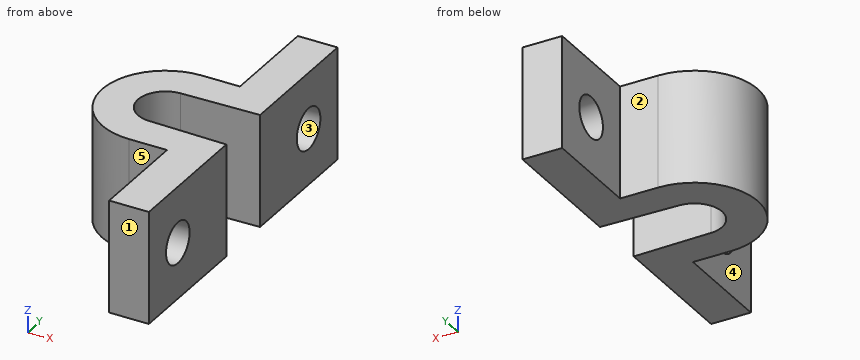
```python
from build123d import *

# Parameters (mm, degrees)
F1_DEPTH = 13
F2_R     = 2.375
F3_DEPTH = 4.6


with BuildPart() as f1:
    # F0 (on Top) → F1 (new body)
    with BuildSketch(Plane.XY):
        with BuildLine():
            Line((-4.6, -19), (0, -19))
            Line((0, -19), (0, -3.4))
            Line((0, -3.4), (-9.075746, -3.184099))
            ThreePointArc((-9.075746, -3.184099), (-12.185, 0), (-9.075746, 3.184099))
            Line((-9.075746, 3.184099), (0, 3.4))
            Line((0, 3.4), (0, 19))
            Line((0, 19), (-4.6, 19))
            Line((-4.6, 19), (-4.6, 7.34))
            Line((-4.6, 7.34), (-9, 7.34))
            ThreePointArc((-9, 7.34), (-16.34, 0), (-9, -7.34))
            Line((-9, -7.34), (-4.6, -7.34))
            Line((-4.6, -7.34), (-4.6, -19))
        make_face()
    extrude(amount=F1_DEPTH)

    # F2 (on Right) → F3 (cut, through all)
    with BuildSketch(Plane.YZ):
        with Locations((-13.17, 6.5)):
            Circle(F2_R)
        with Locations((13.17, 6.5)):
            Circle(F2_R)
    extrude(amount=-F3_DEPTH, mode=Mode.SUBTRACT)


solid = f1.part
```
Model file for the job. Use its own axes, mm. Face numbers are marked on the shaded views. A direction names the side the tool comes from. Give positions to 0.01 mm unless a question says otherwise; leave off trailing zeros. Write each loop counter-clockwise with the first axis right and the second up, starting at its lowest first coordinate (ties: lowest second). Pieces come first, ordered by that corner, then holes. Notation, with made-up numbers: (78.25, -10) -> (94.25, -10) arc R9 cw to (94.25, 4) -> close; hole circle Ø9 at (82.5, 73). An arc over 180 degrees is marked (long way). Use CSV: the item, a comma, the result in double quotes. Start each with the question number.
1) Pin check, flat tips, straight feed: P1, Ø1.3, axis at x = -6, z = 7.5, coming from the +Y side; P2, Ø4, axis at x = -7, z = 7, coming from the -Y side; P3, Ø5.5, axis at y = -13.17, z = 6.5, coming from the -X side. Stop position of each tip, or through.
2) Tool access for the marked faces 1 and 2: list every direction of +Z, -Z, +X, -X, +Y, -Y with a clear straight run to the whole face (end or side of a thin tool).
3) Cut at B-B on y = -13.17. List the corners of the cut face in (x, z) (3 decimals), plus the area to 4 significant figures.
4) Two-plate mould, pull along Y, no slides. Class the marked faces 3, 4 and 5: released by +Y, released by -Y, zero draft, split by the parting line, or undercut.
5) Cut at D-D on z = 3.25. List the corners of the cut face in (x, y) (3 decimals), plus the area to 3 significant figures.
6) Drill centre lines: L1, parallel to Y at x = -4.5, z = 5; L2, parallel to Z at x = -1.75, y = 13.17 (3 decimals); L3, parallel to Y at x = -1.25, z = 5.25. Where is each one in solid material? Low to high.
7) Cut at A-A on z = 6.5. List the corners of the cut face in (x, y) (3 decimals).
8) Cut at C-C on x = -5. List the corners of the cut face in (y, z), plus the area to 3 significant figures.
Final values:
1,P1,"stops at y = 7.34"
1,P2,"stops at y = -7.34"
1,P3,"stops at x = -4.6"
2,face 1,"+Z, -Z, +X, -X, -Y"
2,face 2,"+Z, -Z, -X, +Y"
3,outline,"(-4.6, 0) -> (0, 0) -> (0, 4.125) -> (-4.6, 4.125) -> close; (-4.6, 8.875) -> (0, 8.875) -> (0, 13) -> (-4.6, 13) -> close"
3,area,"37.95 mm2"
4,face 3,"undercut"
4,face 4,"zero draft"
4,face 5,"released by -Y"
5,outline,"(-9.076, -3.184) arc R3.185 cw to (-9.076, 3.184) -> (0, 3.4) -> (0, 19) -> (-4.6, 19) -> (-4.6, 7.34) -> (-9, 7.34) arc R7.34 ccw to (-9, -7.34) -> (-4.6, -7.34) -> (-4.6, -19) -> (0, -19) -> (0, -3.4) -> close"
5,area,"249 mm2"
6,L1,"y = -19 to -15.01, -11.33 to -3.29, 3.29 to 11.33, 15.01 to 19"
6,L2,"z = 0 to 4.125, 8.875 to 13"
6,L3,"y = -19 to -15.19, -11.15 to -3.37, 3.37 to 11.15, 15.19 to 19"
7,outline,"(-9.076, -3.184) arc R3.185 cw to (-9.076, 3.184) -> (0, 3.4) -> (0, 10.795) -> (-4.6, 10.795) -> (-4.6, 7.34) -> (-9, 7.34) arc R7.34 ccw to (-9, -7.34) -> (-4.6, -7.34) -> (-4.6, -10.795) -> (0, -10.795) -> (0, -3.4) -> close; (-4.6, -19) -> (0, -19) -> (0, -15.545) -> (-4.6, -15.545) -> close; (-4.6, 15.545) -> (0, 15.545) -> (0, 19) -> (-4.6, 19) -> close"
8,outline,"(-7.34, 0) -> (-3.28, 0) -> (-3.28, 13) -> (-7.34, 13) -> close; (3.28, 0) -> (7.34, 0) -> (7.34, 13) -> (3.28, 13) -> close"
8,area,"106 mm2"
